```python
from build123d import *

# Parameters (mm, degrees)
SZKIC2_R                    = 5
DODANIE_WYCI_GNI_CIE1_DEPTH = 20
SZKIC2_3_W                  = 15
SZKIC2_3_H                  = 15
DODANIE_WYCI_GNI_CIE2_DEPTH = 10


with BuildPart() as part:
    # Szkic2 → Dodanie-wyci_gni_cie1 (new body)
    with BuildSketch(Plane(origin=(0, 0, 0), x_dir=(1, 0, 0), z_dir=(0, 1, 0))):
        Circle(SZKIC2_R)
    extrude(amount=DODANIE_WYCI_GNI_CIE1_DEPTH)

    # Szkic2_3 → Dodanie-wyci_gni_cie2 (add)
    with BuildSketch(Plane(origin=(0, 0, 0), x_dir=(1, 0, 0), z_dir=(0, 1, 0))):
        Rectangle(SZKIC2_3_W, SZKIC2_3_H)
    extrude(amount=DODANIE_WYCI_GNI_CIE2_DEPTH)


solid = part.part
```
Model file for the job. Use its own axes, mm. A direction names the side the tool comes from. Coordinates: 2 decimals unless noted, no trailing zeros. Loops run counter-clockwise (first coordinate to the right, second up) from the corner with the lowest first, then second, coordinate; pieces in that order, holes last. Notation, with made-up numbers: (-31.75, 85) -> (-16.75, 85) arc R28 cw to (-16.75, 122) -> close; hole circle Ø9 at (64, -7.75). An arc over 180 degrees is marked (long way). Answer as a JSON object with one key per item and string values.
Q1. Cut at B-B (x = 0). List the corners of the cut face in (y, z).
Report:
{"outline": "(0, -7.5) -> (10, -7.5) -> (10, -5) -> (20, -5) -> (20, 5) -> (10, 5) -> (10, 7.5) -> (0, 7.5) -> close"}
Q2. Flat gauge pins, fed straight in: P1, Ø8, axis at y = 18, z = 2.5, coming from the +X side; P2, Ø1, axis at y = 11.5, z = 1.5, coming from the -X side; P3, Ø8, axis at y = 14.5, z = -0.5, coming from the -X side. Where does each tip first touch, or does it go through?
Report:
{"P1": "stops at x = 5", "P2": "stops at x = -4.9", "P3": "stops at x = -5"}
Q3. Probe probe 1 along Y at (x, z) = (-1, 5); probe 2 along Z at (x, y) = (0, 11.25); probe 3 along Z at (x, y) = (-1.75, 11.75). List the from-to ranges inside material, lowest first.
Report:
{"probe 1": "y = 0 to 10", "probe 2": "z = -5 to 5", "probe 3": "z = -4.68 to 4.68"}
Q4. Cut at A-A (z = -4). List the corners of the cut face in (x, y), and give its area (3 significant figures).
Report:
{"outline": "(-7.5, 0) -> (7.5, 0) -> (7.5, 10) -> (3, 10) -> (3, 20) -> (-3, 20) -> (-3, 10) -> (-7.5, 10) -> close", "area": "210 mm2"}
Q5. Cut at D-D (z = 6.75). List the corners of the cut face in (x, y), and give its area (3 significant figures).
Report:
{"outline": "(-7.5, 0) -> (7.5, 0) -> (7.5, 10) -> (-7.5, 10) -> close", "area": "150 mm2"}
Q6. Cut at C-C (x = -6.5). List the corners of the cut face in (y, z).
Report:
{"outline": "(0, -7.5) -> (10, -7.5) -> (10, 7.5) -> (0, 7.5) -> close"}
Q7. 3-axis set-ups, long thin cutter, end or side, ignore diameter. For faces 1 (the flat face through (0, 0, 0)), 2 (the flat face through (-2, 10, -5)): which of +Z, -Z, +X, -X, +Y, -Y reach the whole face in a straight line?
Report:
{"face 1": "+Z, -Z, +X, -X, -Y", "face 2": "+Y"}
